from build123d import *

# Parameters (mm, degrees)
SKETCH1_W           = 60
SKETCH1_H           = 50
BOSS_EXTRUDE1_DEPTH = 50
CUT_EXTRUDE1_DEPTH  = 50
SKETCH3_W           = 60
SKETCH3_H           = 30
CUT_EXTRUDE2_DEPTH  = 30
BOSS_EXTRUDE2_DEPTH = 30
SKETCH9_W           = 60
SKETCH9_H           = 50
CUT_EXTRUDE3_DEPTH  = 10
SKETCH10_W          = 60
SKETCH10_H          = 30
CUT_EXTRUDE4_DEPTH  = 10
BOSS_EXTRUDE7_DEPTH = 30
CUT_EXTRUDE10_DEPTH = 30
SKETCH20_W          = 60
SKETCH20_H          = 42.426406872
CUT_EXTRUDE11_DEPTH = 30


with BuildPart() as part:
    # Sketch1 → Boss-Extrude1 (new body)
    with BuildSketch(Plane.XY):
        with Locations((30, 25)):
            Rectangle(SKETCH1_W, SKETCH1_H)
    extrude(amount=BOSS_EXTRUDE1_DEPTH)

    # Sketch2 → Cut-Extrude1 (cut)
    with BuildSketch(Plane.XZ):
        Polygon((0, 30), (20, 50), (0, 50), align=None)
    extrude(amount=-CUT_EXTRUDE1_DEPTH, mode=Mode.SUBTRACT)

    # Sketch3 → Cut-Extrude2 (cut)
    with BuildSketch(Plane.XY.offset(50)):
        with Locations((30, 35)):
            Rectangle(SKETCH3_W, SKETCH3_H)
    extrude(amount=-CUT_EXTRUDE2_DEPTH, mode=Mode.SUBTRACT)

    # Sketch4 → Boss-Extrude2 (add)
    with BuildSketch(Plane(origin=(0, 35, 35), x_dir=(1, 0, 0), z_dir=(0, 0.707106781, 0.707106781))):
        Polygon((60, -21.213203436), (60, 21.213203436), (0, 21.213203436), (20, -21.213203436), align=None)
    extrude(amount=-BOSS_EXTRUDE2_DEPTH)

    # Sketch9 → Cut-Extrude3 (cut)
    with BuildSketch(Plane(origin=(0, 0, 0), x_dir=(-1, 0, 0), z_dir=(0, 0, -1))):
        with Locations((-30, 25)):
            Rectangle(SKETCH9_W, SKETCH9_H)
    extrude(amount=CUT_EXTRUDE3_DEPTH, mode=Mode.SUBTRACT)

    # Sketch10 → Cut-Extrude4 (cut)
    with BuildSketch(Plane.XZ):
        with Locations((30, 15)):
            Rectangle(SKETCH10_W, SKETCH10_H)
    extrude(amount=CUT_EXTRUDE4_DEPTH, mode=Mode.SUBTRACT)

    # Sketch18 → Boss-Extrude7 (add)
    with BuildSketch(Plane(origin=(0, 20, 0), x_dir=(1, 0, 0), z_dir=(0, 1, 0))):
        Polygon((10, -20), (0, -20), (0, -30), (20, -50), align=None)
    extrude(amount=BOSS_EXTRUDE7_DEPTH)

    # Sketch19 → Cut-Extrude10 (cut)
    with BuildSketch(Plane(origin=(3, 0, -1), x_dir=(-0.316227766, 0, -0.948683298), z_dir=(0.948683298, 0, -0.316227766))):
        Polygon((-22.135943621, 50), (-53.758720223, 20), (-53.758720223, 50), align=None)
    extrude(amount=-CUT_EXTRUDE10_DEPTH, mode=Mode.SUBTRACT)

    # Sketch20 → Cut-Extrude11 (cut)
    with BuildSketch(Plane(origin=(0, 35, 35), x_dir=(1, 0, 0), z_dir=(0, 0.707106781, 0.707106781))):
        with Locations((30, 0)):
            Rectangle(SKETCH20_W, SKETCH20_H)
    extrude(amount=CUT_EXTRUDE11_DEPTH, mode=Mode.SUBTRACT)


solid = part.part
Can you work these out from the model? Positions are in its coordinate system, mm. Coordinates: 2 decimals unless noted, no trailing zeros. Write each loop counter-clockwise with the first axis right and the second up, starting at its lowest first coordinate (ties: lowest second). Pieces come first, ordered by that corner, then holes.
Q1. Please list where these lines run through material, in increasing order: L1, parallel to Y at x = 17, z = 40; L2, parallel to Z at x = 54.5, y = 44; L3, parallel to Z at x = 14, y = 24.
Results found:
L1: y = 0 to 30
L2: z = 0 to 26
L3: z = 0 to 44
Q2. Imagine slicing it at B-B, the plane x = 53. List the corners of the cut face in (y, z) for me, plus the area to 3 significant figures.
Results found:
outline: (0, 0) - (50, 0) - (50, 20) - (20, 50) - (0, 50) - close
area: 2,050 mm2
Q3. For P1, Ø5, axis at x = 11.5, z = 22.5, coming from the -Y side; P2, Ø4, axis at x = 11, y = 15, coming from the +Z side; P3, Ø1.5, axis at y = 19, z = 38, coming from the -X side; P4, Ø12, axis at x = 19.5, z = 31.5, coming from the +Y side, each with a flat end and sliding along its axis, tell me the tip position at first contact or that it passes through.
Results found:
P1: stops at y = 0
P2: stops at z = 43
P3: stops at x = 7.25
P4: stops at y = 44.5
Q4. Imagine slicing it at C-C, the plane z = 33.5. List the corners of the cut face in (x, y) for me, plus the area to 3 significant figures.
Results found:
outline: (3.5, 0) - (60, 0) - (60, 36.5) - (3.5, 36.5) - close
area: 2,060 mm2
Q5. Imagine slicing it at D-D, the plane y = 45.5. List the corners of the cut face in (x, z) for me.
Results found:
outline: (0, 0) - (60, 0) - (60, 24.5) - (0, 24.5) - close
Q6. Imagine slicing it at A-A, the plane y = 22.5. List the corners of the cut face in (x, z) for me.
Results found:
outline: (0, 0) - (60, 0) - (60, 47.5) - (17.5, 47.5) - (0, 30) - close
